Source: CAD feature listing. Evaluate the final solid. Frame: model axes, mm. Give positions to 0.01 mm unless a question says otherwise; leave off trailing zeros. Write each loop counter-clockwise with the first axis right and the second up, starting at its lowest first coordinate (ties: lowest second). Pieces come first, ordered by that corner, then holes. Notation, with made-up numbers: (-35.5, -17.75) -> (0.5, -17.75) arc R35 ccw to (0.5, 14.25) -> close; hole circle Ø11 at (-11, -32.5). An arc over 180 degrees is marked (long way). Write item = value, one per line.
from build123d import *

# Parameters (mm, degrees)
CROQUIS1_R              = 1.9
SALIENTE_EXTRUIR1_DEPTH = 5.25
CHAFL_N1_SIZE           = 1.5


with BuildPart() as part:
    # Croquis1 → Saliente-Extruir1 (new body)
    with BuildSketch(Plane(origin=(0, 0, 0), x_dir=(1, 0, 0), z_dir=(0, 1, 0))):
        with BuildLine():
            Line((34.209401077, 5.5), (-34.209401077, 5.5))
            ThreePointArc((-34.209401077, 5.5), (-35.623614639, 4.914213562), (-36.209401077, 3.5))
            Line((-36.209401077, 3.5), (-36.209401077, -1.75))
            ThreePointArc((-36.209401077, -1.75), (-35.623614639, -3.164213562), (-34.209401077, -3.75))
            Line((-34.209401077, -3.75), (34.209401077, -3.75))
            ThreePointArc((34.209401077, -3.75), (35.623614639, -3.164213562), (36.209401077, -1.75))
            Line((36.209401077, -1.75), (36.209401077, 3.5))
            ThreePointArc((36.209401077, 3.5), (35.623614639, 4.914213562), (34.209401077, 5.5))
        make_face()
        with Locations(Location((29.498076211, 0, 0), (0, 0, 90))):
            Circle(CROQUIS1_R, mode=Mode.SUBTRACT)
        with Locations(Location((14.748076211, 0, 0), (0, 0, 90))):
            Circle(CROQUIS1_R, mode=Mode.SUBTRACT)
        with Locations(Location((0, 0, 0), (0, 0, 90))):
            Circle(CROQUIS1_R, mode=Mode.SUBTRACT)
        with Locations(Location((-14.748076211, 0, 0), (0, 0, 90))):
            Circle(CROQUIS1_R, mode=Mode.SUBTRACT)
        with Locations(Location((-29.498076211, 0, 0), (0, 0, 90))):
            Circle(CROQUIS1_R, mode=Mode.SUBTRACT)
    extrude(amount=SALIENTE_EXTRUIR1_DEPTH)

    # Chaflán1
    # the kernel refuses this chamfer: 1.5 mm, written as the material it takes off along each edge
    with BuildSketch(Plane(origin=(38.066925559, 5.25, -5.5), x_dir=(0, -0.9996219169112969, -0.027495876610586202), z_dir=(-1, 0, 0))) as chafl_n1_piece_1:
        Polygon((CHAFL_N1_SIZE * 0.999621916911, CHAFL_N1_SIZE * 0.0274958766106), (-CHAFL_N1_SIZE * 0.0274958766106, CHAFL_N1_SIZE * 0.999621916911), (0, 0), align=None)
    extrude(amount=76.133851117, mode=Mode.SUBTRACT)


solid = part.part
(1) Material intervals for line 1 (X direction, y = 1.65, z = 0); line 2 (X direction, y = 2.6, z = -1.25); line 3 (Z direction, x = 15, y = 3.05), sorted ascending.
Values follow:
line_1 = -36.21 to -31.4, -27.6 to -16.65, -12.85 to -1.9, 1.9 to 12.85, 16.65 to 27.6, 31.4 to 36.21
line_2 = -36.21 to -30.93, -28.07 to -16.18, -13.32 to -1.43, 1.43 to 13.32, 16.18 to 28.07, 30.93 to 36.21
line_3 = -5.5 to -1.88, 1.88 to 3.75
(2) Section query A-A (z = 0). Return loops of the section in (x, y).
Values follow:
outline = (-36.21, 0) -> (-31.4, 0) -> (-31.4, 5.25) -> (-36.21, 5.25) -> close; (-27.6, 0) -> (-16.65, 0) -> (-16.65, 5.25) -> (-27.6, 5.25) -> close; (-12.85, 0) -> (-1.9, 0) -> (-1.9, 5.25) -> (-12.85, 5.25) -> close; (1.9, 0) -> (12.85, 0) -> (12.85, 5.25) -> (1.9, 5.25) -> close; (16.65, 0) -> (27.6, 0) -> (27.6, 5.25) -> (16.65, 5.25) -> close; (31.4, 0) -> (36.21, 0) -> (36.21, 5.25) -> (31.4, 5.25) -> close
(3) Pull-direction query (Z, two-part tool) for faces 1 (the face through (36.209, 3, -1)), 2 (the face through (0.728, 2.588, -1.755)), 3 (the face through (-35.64, 2.59, 3.15)); classes: pulls with the +Z half, pulls with the -Z half, needs draft (parallel to the pull), parting line crosses it, or undercut.
Values follow:
face_1 = needs draft
face_2 = undercut
face_3 = pulls with the +Z half
(4) Section query C-C (y = 1.7). Return loops of the section in (x, z).
Values follow:
outline = (-36.21, -3.5) arc R2 ccw to (-34.21, -5.5) -> (34.21, -5.5) arc R2 ccw to (36.21, -3.5) -> (36.21, 1.75) arc R2 ccw to (34.21, 3.75) -> (-34.21, 3.75) arc R2 ccw to (-36.21, 1.75) -> close; hole circle Ø3.8 at (-29.5, 0); hole circle Ø3.8 at (-14.75, 0); hole circle Ø3.8 at (0, 0); hole circle Ø3.8 at (14.75, 0); hole circle Ø3.8 at (29.5, 0)
(5) First-contact query: pin 1 (5 mm diameter, centred on x = 0, z = 0, fed in from -Y). Flat tip, straight axial feed; report the tip coordinate or a pass-through.
Values follow:
pin_1 = 0
(6) Section query B-B (x = 0). Return loops of the section in (y, z), plus the area to 3 significant figures.
Values follow:
outline = (0, -5.5) -> (3.75, -5.5) -> (5.25, -4) -> (5.25, -1.9) -> (0, -1.9) -> close; (0, 1.9) -> (5.25, 1.9) -> (5.25, 3.75) -> (0, 3.75) -> close
area = 27.5 mm2
(7) Section query D-D (x = -9.5). Return loops of the section in (y, z), plus the area to 3 significant figures.
Values follow:
outline = (0, -5.5) -> (3.75, -5.5) -> (5.25, -4) -> (5.25, 3.75) -> (0, 3.75) -> close
area = 47.4 mm2
